The listing builds one solid part. Answer for the finished solid, in the listing's coordinates (mm). A direction names the side the tool comes from. Give positions to 0.01 mm unless a question says otherwise; leave off trailing zeros. Loops run counter-clockwise (first coordinate to the right, second up) from the corner with the lowest first, then second, coordinate; pieces in that order, holes last. Notation, with made-up numbers: (68.5, -36) -> (78.5, -36) arc R31 cw to (78.5, -7) -> close; hole circle Ø1 at (65.5, 32.25). An arc over 180 degrees is marked (long way). One line per question, with ' | ' between items. Start each with the question number.
from build123d import *

# Parameters (mm, degrees)
SKETCH_1_W          = 20
SKETCH_1_H          = 20
SKETCH_1_W_2        = 18
SKETCH_1_H_2        = 18
EXTRUDE_1_DEPTH     = 135
SKETCH_2_R          = 1.5
CUT_EXTRUDE_1_DEPTH = 100


with BuildPart() as part:
    # 草图1 → 凸台-拉伸1 (new, symmetric)
    with BuildSketch(Plane.XY):
        Rectangle(SKETCH_1_W, SKETCH_1_H)
        Rectangle(SKETCH_1_W_2, SKETCH_1_H_2, mode=Mode.SUBTRACT)
    extrude(amount=EXTRUDE_1_DEPTH, both=True)

    # 草图2 → 切除-拉伸1 (cut)
    with BuildSketch(Plane(origin=(0, 10, 0), x_dir=(1, 0, 0), z_dir=(0, 1, 0))):
        with Locations(Location((0, -125, 0), (0, 0, 270))):
            Circle(SKETCH_2_R)
        with Locations(Location((0, -115, 0), (0, 0, 270))):
            Circle(SKETCH_2_R)
        with Locations(Location((0, -105, 0), (0, 0, 270))):
            Circle(SKETCH_2_R)
    extrude(amount=-CUT_EXTRUDE_1_DEPTH, mode=Mode.SUBTRACT)


solid = part.part
1. For faces 4 (the flat face through (-0.8, -9.6, -135)), 5 (the flat face through (0, -9, 2)), determine the directions among +Z, -Z, +X, -X, +Y, -Y from which every point of the face is accessible in a straight line to the end or side of a thin tool.
2. The part is cut by section A-A (x = 5.5). Write down the section's boundary in (y, z), plus the area to 3 significant figures.
3. The part is cut by section C-C (z = 81.5). Write down the section's boundary in (x, y), plus the area to 3 significant figures.
4. Determine the mould class of faces 1 (the flat face through (0, 10, 2)), 2 (the flat face through (-10, 0, 2)), 3 (the flat face through (-9, 0, 2)) for opening direction Y: released by +Y, released by -Y, zero draft, split by the parting line, or undercut.
5. This flat-tipped pin is pushed along its axis until it touches: pin 1 Ø5 at (x, z) = (0, 115) entering from +Y. Where does it stop, or does it pass through?
6. Straight lines are drawn through the part: L1, parallel to Y at x = -8.5, z = -112.5; L2, parallel to X at y = -9.4, z = 115. For each, find the intervals that lie inside material, in ascending order.
Check sheet entries:
1) face 4: -Z, +X, -X, +Y, -Y | face 5: +Z, -Z
2) outline: (-10, -135) -> (-9, -135) -> (-9, 135) -> (-10, 135) -> close; (9, -135) -> (10, -135) -> (10, 135) -> (9, 135) -> close | area: 540 mm^2
3) outline: (-10, -10) -> (10, -10) -> (10, 10) -> (-10, 10) -> close; hole (-9, -9) -> (9, -9) -> (9, 9) -> (-9, 9) -> close | area: 76.0 mm^2
4) face 1: released by +Y | face 2: zero draft | face 3: undercut
5) pin 1: stops at y = 10
6) L1: y = -10 to -9, 9 to 10 | L2: x = -10 to -1.5, 1.5 to 10
